Design review of the part built by this model. Coordinates are the model's own, in mm. A direction names the side the tool comes from. Give positions to 0.01 mm unless a question says otherwise; leave off trailing zeros. Write each loop counter-clockwise with the first axis right and the second up, starting at its lowest first coordinate (ties: lowest second). Pieces come first, ordered by that corner, then holes. Notation, with made-up numbers: M -13.75,36.5 L 29.25,36.5 A27 cw 29.25,53.5 Z; hole C 78,53.5 d5. An arc over 180 degrees is marked long. Answer in a Markdown table with one row per item.
Autodesk Inventor part; units mm, degrees
ref_plane "YZ Plane" through (0, 0, 0) normal (1, 0, 0) x (0, 1, 0)
ref_plane "XZ Plane" through (0, 0, 0) normal (0, 1, 0) x (-1, 0, 0)
ref_plane "XY Plane" through (0, 0, 0) normal (0, 0, 1) x (1, 0, 0)
sketch "Sketch1" plane through (0, 0, 0) normal (0, 0, 1) x (1, 0, 0)
  line L0 (0, 0) -> (126.85, 0)
  line L1 (126.85, 0) -> (126.85, 64.605)
  line L2 (126.85, 64.605) -> (0, 64.605)
  line L3 (0, 64.605) -> (0, 0)
  line L4 (55.925, 0) -> (65.5708, 0)
  line L5 (53.975, 0) -> (72.875, 0)
  line L6 (72.875, 0) -> (72.875, 39.5)
  line L7 (72.875, 39.5) -> (53.975, 39.5)
  line L8 (53.975, 39.5) -> (53.975, 0)
  line L9 (51.975, 0) -> (74.875, 0)
  line L10 (74.875, 0) -> (74.875, 41.5)
  line L11 (74.875, 41.5) -> (51.975, 41.5)
  line L12 (51.975, 41.5) -> (51.975, 0)
  point P0 (74.875, 20.75)
  point P1 (74.875, 0)
  dimension "d0" = 126.85
  dimension "d1" = 64.605
  dimension "d3" = 39.5
  dimension "d4" = 18.9
  dimension "d5" = 53.975
  dimension "d6" = 2
  dimension "d7" = 2
  dimension "d8" = 2
extrude "Extrusion2" add sketch "Sketch1" along normal blind 5.235 contours L3 L2 L1 L0 L10 L11 L12
extrude "Extrusion3" add sketch "Sketch1" along normal blind 8.235 contours L12 L11 L10 L0 L6 L7 L8
extrude "Extrusion4" add sketch "Sketch1" along normal blind 5.235 contours L8 L7 L6 L0
sketch "Sketch2" plane through (0, 0, 8.235) normal (0, 0, 1) x (1, 0, 0)
  line L0 (72.875, 39.5) -> (72.875, 0)
  line L1 (72.875, 0) -> (74.875, 0)
  line L2 (74.875, 0) -> (74.875, 41.5)
  line L3 (74.875, 41.5) -> (51.975, 41.5)
  line L4 (51.975, 41.5) -> (51.975, 0)
  line L5 (51.975, 0) -> (53.975, 0)
  line L6 (53.975, 0) -> (53.975, 39.5)
  line L7 (53.975, 39.5) -> (72.875, 39.5)
  line L8 (51.975, 0) -> (53.975, 0)
  line L9 (53.975, 0) -> (53.975, 2.5)
  line L10 (53.975, 2.5) -> (51.975, 2.5)
  line L11 (51.975, 2.5) -> (51.975, 0)
  line L12 (72.875, 0) -> (74.875, 0)
  line L13 (74.875, 0) -> (74.875, 2.5)
  line L14 (74.875, 2.5) -> (72.875, 2.5)
  line L15 (72.875, 2.5) -> (72.875, 0)
  point P0 (0, 0)
  dimension "d17" = 2.5
  dimension "d18" = 2.5
extrude "Extrusion5" cut sketch "Sketch2" against normal blind 3 contours L14 L2 L1 L0 | L6 L5 L4 L10
fillet "Fillet1" radius 2.5 4 edges at (126.85, 0, 2.6175) (0, 0, 2.6175) (126.85, 64.605, 2.6175) (0, 64.605, 2.6175)
sketch "Sketch3" plane through (0, 0, 5.235) normal (0, 0, 1) x (1, 0, 0)
  line L0 (0, 0) -> (15, 0)
  line L1 (15, 0) -> (15, 15)
  line L2 (15, 15) -> (0, 15)
  line L3 (0, 15) -> (0, 0)
  line L4 (0, 64.605) -> (15, 64.605)
  line L5 (15, 64.605) -> (15, 49.605)
  line L6 (15, 49.605) -> (0, 49.605)
  line L7 (0, 49.605) -> (0, 64.605)
  line L8 (124.35, 0) -> (2.5, 0)
  line L9 (126.85, 2.5) -> (126.85, 62.105)
  line L10 (126.85, 15) -> (111.85, 15)
  line L11 (111.85, 15) -> (111.85, 0)
  line L12 (111.85, 0) -> (126.85, 0)
  line L13 (126.85, 0) -> (126.85, 15)
  line L14 (126.85, 64.605) -> (111.85, 64.605)
  line L15 (111.85, 64.605) -> (111.85, 49.605)
  line L16 (111.85, 49.605) -> (126.85, 49.605)
  line L17 (126.85, 49.605) -> (126.85, 64.605)
  circle A0 centre (7.5, 57.44) radius 2.15
  circle A1 centre (119.35, 57.44) radius 2.15
  circle A2 centre (119.35, 7.165) radius 2.15
  line L18 (0, 62.105) -> (0, 2.5)
  circle A3 centre (7.5, 7.165) radius 2.15
  point P0 (111.85, 7.5)
  point P1 (119.35, 0)
  point P2 (119.35, 15)
  point P3 (7.5, 64.605)
  dimension "d22" = 15
  dimension "d23" = 15
  dimension "d24" = 15
  dimension "d25" = 15
  dimension "d26" = 64.605
  dimension "d28" = 15
  dimension "d29" = 15
  dimension "d30" = 15
  dimension "d31" = 15
  dimension "d32" = 64.605
  dimension "d33" = 0
  dimension "d52" = 7.165
  dimension "d53" = 7.5
  dimension "d54" = 4.3
  dimension "d55" = 4.3
  dimension "d56" = 7.5
  dimension "d57" = 7.165
  dimension "d58" = 4.3
  dimension "d59" = 7.5
  dimension "d61" = 7.165
  dimension "d62" = 0
  dimension "d63" = 4.3
  dimension "d65" = 7.5
  dimension "d66" = 7.165
sketch "Sketch4" plane through (0, 0, 0) normal (0, 0, -1) x (-1, 0, 0)
  line L0 (-126.85, 0) -> (-111.85, 0)
  line L1 (-111.85, 0) -> (-111.85, 15)
  line L2 (-111.85, 15) -> (-126.85, 15)
  line L3 (-126.85, 15) -> (-126.85, 0)
  line L4 (-126.85, 64.605) -> (-111.85, 64.605)
  line L5 (-111.85, 64.605) -> (-111.85, 49.605)
  line L6 (-111.85, 49.605) -> (-126.85, 49.605)
  line L7 (-126.85, 49.605) -> (-126.85, 64.605)
  line L8 (-85.2582, 0) -> (-207.1082, 0)
  line L9 (0, -43.3004) -> (0, 16.3046)
  line L10 (0, 15) -> (-15, 15)
  line L11 (-15, 15) -> (-15, 0)
  line L12 (-15, 0) -> (0, 0)
  line L13 (0, 0) -> (0, 15)
  line L14 (0, 64.605) -> (-15, 64.605)
  line L15 (-15, 64.605) -> (-15, 49.605)
  line L16 (-15, 49.605) -> (0, 49.605)
  line L17 (0, 49.605) -> (0, 64.605)
  line L18 (-2.5, 0) -> (-124.35, 0)
  line L19 (0, 62.105) -> (0, 2.5)
  line L20 (-126.85, 2.5) -> (-126.85, 62.105)
  point P0 (0, 0)
  point P1 (-15, 7.5)
  point P2 (-7.5, 0)
  point P3 (-7.5, 15)
  point P4 (0, 32.3025)
  point P5 (-119.35, 0)
  dimension "d34" = 15
  dimension "d35" = 15
  dimension "d36" = 15
  dimension "d37" = 15
  dimension "d38" = 64.605
  dimension "d39" = 0
  dimension "d40" = 15
  dimension "d41" = 15
  dimension "d42" = 15
  dimension "d43" = 15
  dimension "d44" = 64.605
  dimension "d45" = 0
  dimension "d46" = 0
  dimension "d47" = 0
  dimension "d48" = 0
  dimension "d49" = 0
extrude "Extrusion7" cut sketch "Sketch3" against normal blind 3.235 contours A0 | A1 | A2 | A3
sketch "Sketch5" plane through (0, 0, 0) normal (0, 0, -1) x (-1, 0, 0)
  circle A0 centre (-7.5, 7.165) radius 2.15
  circle A1 centre (-7.5, 57.44) radius 2.15
  circle A2 centre (-119.35, 57.44) radius 2.15
  circle A3 centre (-119.35, 7.165) radius 2.15
  circle A4 centre (-7.5, 7.165) radius 4
  circle A5 centre (-119.35, 7.165) radius 4
  circle A6 centre (-119.35, 57.44) radius 4
  circle A7 centre (-7.5, 57.44) radius 4
  point P0 (0, 0)
  dimension "d69" = 8
  dimension "d70" = 8
  dimension "d71" = 8
  dimension "d72" = 8
sketch "Sketch6" plane through (0, 0, 5.235) normal (0, 0, 1) x (1, 0, 0)
  line L0 (126.85, 2.5) -> (126.85, 62.105)
  circle A0 centre (119.35, 57.44) radius 2.15
  circle A1 centre (7.5, 7.165) radius 2.15
  circle A2 centre (119.35, 7.165) radius 2.15
  circle A3 centre (7.5, 57.44) radius 2.15
  arc A4 (2.5, 64.605) -> (0, 62.105) centre (2.5, 62.105) ccw
  line L1 (0, 62.105) -> (0, 2.5)
  arc A5 (0, 2.5) -> (2.5, 0) centre (2.5, 2.5) ccw
  line L2 (124.35, 0) -> (2.5, 0)
  arc A6 (124.35, 0) -> (126.85, 2.5) centre (124.35, 2.5) ccw
  line L3 (126.85, 2.5) -> (126.85, 62.105)
  arc A7 (126.85, 62.105) -> (124.35, 64.605) centre (124.35, 62.105) ccw
  line L4 (124.35, 64.605) -> (2.5, 64.605)
  line L5 (72.875, 2.5) -> (74.875, 2.5)
  line L6 (72.875, 39.5) -> (72.875, 2.5)
  line L7 (53.975, 39.5) -> (72.875, 39.5)
  line L8 (53.975, 2.5) -> (53.975, 39.5)
  line L9 (51.975, 2.5) -> (53.975, 2.5)
  line L10 (51.975, 2.5) -> (51.975, 41.5)
  line L11 (51.975, 41.5) -> (74.875, 41.5)
  line L12 (74.875, 41.5) -> (74.875, 2.5)
  line L13 (72.875, 2.5) -> (74.875, 2.5)
  line L14 (74.875, 2.5) -> (74.875, 41.5)
  line L15 (74.875, 41.5) -> (51.975, 41.5)
  line L16 (51.975, 41.5) -> (51.975, 2.5)
  line L17 (51.975, 2.5) -> (53.975, 2.5)
  line L18 (53.975, 2.5) -> (53.975, 39.5)
  line L19 (53.975, 39.5) -> (72.875, 39.5)
  line L20 (72.875, 39.5) -> (72.875, 2.5)
  point P0 (0, 0)
sketch "Sketch7" plane through (0, 0, 8.235) normal (0, 0, 1) x (1, 0, 0)
  line L0 (72.875, 2.5) -> (74.875, 2.5)
  line L1 (74.875, 2.5) -> (74.875, 41.5)
  line L2 (74.875, 41.5) -> (51.975, 41.5)
  line L3 (51.975, 41.5) -> (51.975, 2.5)
  line L4 (51.975, 2.5) -> (53.975, 2.5)
  line L5 (53.975, 2.5) -> (53.975, 39.5)
  line L6 (53.975, 39.5) -> (72.875, 39.5)
  line L7 (72.875, 39.5) -> (72.875, 2.5)
  point P0 (0, 0)
extrude "Extrusion8" add sketch "Sketch7" along normal blind 3
extrude "Extrusion9" add sketch "Sketch6" along normal blind 3
extrude "Extrusion10" cut sketch "Sketch5" against normal blind 5
extrude "Extrusion11" cut sketch "Sketch5" against normal blind 10 contours A0 | A1 | A2 | A3
properties part number "KeypadBase"
1) Add section C-C (y = 34.5). Write out the cut boundary in (x, z) (3 decimals), and give its area (3 significant figures).
Geometry says:
| item | result |
|---|---|
| outline | M 0,0 L 126.85,0 L 126.85,8.235 L 74.875,8.235 L 74.875,11.235 L 72.875,11.235 L 72.875,8.235 L 53.975,8.235 L 53.975,11.235 L 51.975,11.235 L 51.975,8.235 L 0,8.235 Z |
| area | 1,060 mm^2 |
2) Add section B-B (x = 7.5). Write out the cut boundary in (y, z) (3 decimals).
Geometry says:
| item | result |
|---|---|
| outline | M 0,0 L 3.165,0 L 3.165,5 L 5.015,5 L 5.015,8.235 L 0,8.235 Z; M 9.315,5 L 11.165,5 L 11.165,0 L 53.44,0 L 53.44,5 L 55.29,5 L 55.29,8.235 L 9.315,8.235 Z; M 59.59,5 L 61.44,5 L 61.44,0 L 64.605,0 L 64.605,8.235 L 59.59,8.235 Z |
3) To check wall thickness, follow probe 1 along X at (y, z) = (57.44, 6.4); probe 2 along Y at (x, z) = (119.35, 2.7) (3 decimals); probe 3 along Y at (x, z) = (7.5, 6.3) (3 decimals). State the ranges of each line that lie inside material, in increasing order. Write a range as [from, to].
Geometry says:
| item | result |
|---|---|
| probe 1 | [0, 5.35], [9.65, 117.2], [121.5, 126.85] |
| probe 2 | [0, 3.165], [11.165, 53.44], [61.44, 64.605] |
| probe 3 | [0, 5.015], [9.315, 55.29], [59.59, 64.605] |
4) The part is to be moulded in two halves that separate along X. For faces 6 (the face through (6, 5, 5)), 7 (the face through (64, 41.5, 10)), 8 (the face through (0.752, 0.713, 4.06)), say which applies: released by +X, released by -X, zero draft, split by the parting line, or undercut.
Geometry says:
| item | result |
|---|---|
| face 6 | undercut |
| face 7 | zero draft |
| face 8 | released by -X |
5) For faces 1 (the face through (63, 39.5, 10)), 2 (the face through (10.448, 9.868, 2.465)), 3 (the face through (8.49, 59.35, 6.59)), 4 (the face through (0, 33, 4)), 5 (the face through (74.875, 22, 10)), list the 3-axis set-ups (+Z, -Z, +X, -X, +Y, -Y) from which the entire face can be reached by the end or side of a thin tool; tool diameter is ignored.
Geometry says:
| item | result |
|---|---|
| face 1 | +Z, -Y |
| face 2 | -Z |
| face 3 | +Z, -Z |
| face 4 | +Z, -Z, -X, +Y, -Y |
| face 5 | +Z, +X, +Y, -Y |
6) Insertion check: P1, Ø3.5, axis at y = 14.5, z = 9, coming from the +X side; P2, Ø2, axis at x = 73.5, z = 10, coming from the -Y side; P3, Ø4, axis at x = 9, y = 7, coming from the -Z side; P4, Ø8, axis at x = 98.5, y = 21, coming from the +Z side (3 decimals). Each pin has a flat end and moves straight along its axis. Give the tip position at first contact, or say it passes through.
Geometry says:
| item | result |
|---|---|
| P1 | x = 126.85 |
| P2 | y = 2.5 |
| P3 | z = 5 |
| P4 | z = 8.235 |
7) Add section A-A (y = 57.44). Write out the cut boundary in (x, z) (3 decimals), and give its area (3 significant figures).
Geometry says:
| item | result |
|---|---|
| outline | M 0,0 L 3.5,0 L 3.5,5 L 5.35,5 L 5.35,8.235 L 0,8.235 Z; M 9.65,5 L 11.5,5 L 11.5,0 L 115.35,0 L 115.35,5 L 117.2,5 L 117.2,8.235 L 9.65,8.235 Z; M 121.5,5 L 123.35,5 L 123.35,0 L 126.85,0 L 126.85,8.235 L 121.5,8.235 Z |
| area | 937 mm^2 |
8) Add section D-D (z = 1.75). Write out the cut boundary in (x, y) (3 decimals).
Geometry says:
| item | result |
|---|---|
| outline | M 0,2.5 A2.5 ccw 2.5,0 L 124.35,0 A2.5 ccw 126.85,2.5 L 126.85,62.105 A2.5 ccw 124.35,64.605 L 2.5,64.605 A2.5 ccw 0,62.105 Z; hole C 7.5,7.165 d8; hole C 7.5,57.44 d8; hole C 119.35,7.165 d8; hole C 119.35,57.44 d8 |
